```python
from build123d import *

# Parameters (mm, degrees)
SKETCH1_W                        = 35.042145822
SKETCH1_H                        = 39.6494
BOSS_EXTRUDE1_DEPTH              = 3.175
F_9_64_0_14063_DIAMETER_HOLE1_D  = 3.572002
F_5_64_0_07813_DIAMETER_HOLE1_D  = 1.984502
F_1_8_0_125_DIAMETER_HOLE1_D     = 3.175
F_1_8_0_125_DIAMETER_HOLE1_DEPTH = 1.27
F_1_8_0_125_DIAMETER_HOLE1_TIP   = 0.953866233


with BuildPart() as part:
    # Sketch1 → Boss-Extrude1 (new body)
    with BuildSketch(Plane.XY):
        with Locations((2.821072911, 35.354563982)):
            Rectangle(SKETCH1_W, SKETCH1_H)
    extrude(amount=BOSS_EXTRUDE1_DEPTH)

    # 9/64 (0.14063) Diameter Hole1 (through all)
    with Locations(Plane.XY.offset(3.175)):
        with Locations((13.992145822, 40.434563982)):
            Hole(F_9_64_0_14063_DIAMETER_HOLE1_D / 2)

    # 5/64 (0.07813) Diameter Hole1 (through all)
    with Locations(Plane.XY.offset(3.175)):
        with Locations((-11.525, 40.434563982), (-11.525, 52.004263982), (17.167145822, 52.004263982), (2.821072911, 40.434563982), (-11.525, 30.274563982), (-11.525, 18.704863982), (17.167145822, 18.704863982), (17.167145822, 30.274563982)):
            Hole(F_5_64_0_07813_DIAMETER_HOLE1_D / 2)

    # 1/8 (0.125) Diameter Hole1
    with Locations(Plane.XY.offset(3.175)):
        with Locations((17.167145822, 18.704863982), (-11.525, 18.704863982), (-11.525, 30.274563982), (17.167145822, 30.274563982), (2.821072911, 40.434563982), (-11.525, 40.434563982), (17.167145822, 52.004263982), (-11.525, 52.004263982)):
            Hole(F_1_8_0_125_DIAMETER_HOLE1_D / 2, depth=F_1_8_0_125_DIAMETER_HOLE1_DEPTH)
            with Locations((0, 0, -(F_1_8_0_125_DIAMETER_HOLE1_DEPTH + F_1_8_0_125_DIAMETER_HOLE1_TIP / 2))):  # 118° drill point
                Cone(0, F_1_8_0_125_DIAMETER_HOLE1_D / 2, F_1_8_0_125_DIAMETER_HOLE1_TIP, mode=Mode.SUBTRACT)


solid = part.part
```
Source: CAD feature listing. Evaluate the final solid. Frame: model axes, mm. A direction names the side the tool comes from. Coordinates: 2 decimals unless noted, no trailing zeros. One line per item, written item: value. Start each with the question number.
Q1. Set-up query: faces 5 (the face through (17.898, 19.375, 0.763)), 6 (the face through (-10.355, 31.347, 2.531)). Return all of +Z, -Z, +X, -X, +Y, -Y with unobstructed straight access to the full face (end or side cutting, diameter ignored); none if empty.
Q2. Line query: line 1 along Y through (x, z) = (-11.5, 1.2); line 2 along Y through (x, z) = (17, 2.4); line 3 along Y through (x, z) = (-11, 2.4). Output: solid intervals per line, ascending.
Q3. Contact query for flat-ended pins moving along their axis: P1, Ø2.5, axis at x = 17.17, y = 18.7, coming from the +Z side; P2, Ø3, axis at x = -11.52, y = 30.27, coming from the +Z side; P3, Ø1.6, axis at x = -11.52, y = 52, coming from the +Z side. Output: stop coordinate, or through.
Q4. Section query A-A, the plane z = 2.55. Give the number of separate pieces and of enclosed holes in the cut face, and give its area (3 significant figures).
Q5. Mould query, pull axis X, two halves, no side actions, for faces 1 (the face through (3, 15.53, 2)), 2 (the face through (20.342, 35, 2)), 3 (the face through (-10.265, 39.469, 2.531)), 4 (the face through (-11.4, 19.69, 0.76)). Classes: pulls with the +X half, pulls with the -X half, needs draft (parallel to the pull), parting line crosses it, or undercut.
Results:
1. face 5: +Z, -Z
1. face 6: +Z
2. line 1: 15.53 to 17.71, 19.7 to 29.28, 31.27 to 39.44, 41.43 to 51.01, 53 to 55.18
2. line 2: 15.53 to 17.13, 20.28 to 28.7, 31.85 to 50.43, 53.58 to 55.18
2. line 3: 15.53 to 17.21, 20.2 to 28.78, 31.77 to 38.94, 41.93 to 50.51, 53.5 to 55.18
3. P1: z = 1.71
3. P2: z = 1.86
3. P3: through
4. separate pieces: 1
4. enclosed holes: 9
4. area: 1,320 mm^2
5. face 1: needs draft
5. face 2: pulls with the +X half
5. face 3: undercut
5. face 4: undercut
